```python
from build123d import *

# Parameters (mm, degrees)
SKETCH4_R           = 2.1
BOSS_EXTRUDE3_DEPTH = 1.2
SKETCH5_W           = 84.339489928
SKETCH5_H           = 2
BOSS_EXTRUDE4_DEPTH = 2.4
SKETCH6_R           = 2.1
BOSS_EXTRUDE5_DEPTH = 1.2


with BuildPart() as part:
    # Sketch4 → Boss-Extrude3 (new body)
    with BuildSketch(Plane(origin=(0, 0, 0), x_dir=(1, 0, 0), z_dir=(0, 1, 0))):
        Polygon((39.4127274, 47.640295112), (-2.757017564, 47.640295112), (-2.757017564, 45.640295112), (39.4127274, 0.640295112), align=None)
        with Locations((22.381300815, 25.64100497)):
            Circle(SKETCH4_R, mode=Mode.SUBTRACT)
        Polygon((81.582472364, 47.640295112), (39.4127274, 47.640295112), (39.4127274, 0.640295112), (81.582472364, 45.640295112), align=None)
        with Locations((56.444153985, 25.64100497)):
            Circle(SKETCH4_R, mode=Mode.SUBTRACT)
    extrude(amount=BOSS_EXTRUDE3_DEPTH)

    # Sketch5 → Boss-Extrude4 (add)
    with BuildSketch(Plane(origin=(0, 0, 0), x_dir=(-1, 0, 0), z_dir=(0, -1, 0))):
        with Locations((-39.4127274, 46.640295112)):
            Rectangle(SKETCH5_W, SKETCH5_H)
    extrude(amount=BOSS_EXTRUDE4_DEPTH)

    # Sketch6 → Boss-Extrude5 (add)
    with BuildSketch(Plane(origin=(0, -2.4, 0), x_dir=(-1, 0, 0), z_dir=(0, -1, 0))):
        Polygon((2.757017564, 47.640295112), (-81.582472364, 47.640295112), (-81.582472364, 45.640295112), (-39.4127274, 0.640295112), (2.757017564, 45.640295112), align=None)
        with Locations((-22.381300815, 25.64100497)):
            Circle(SKETCH6_R, mode=Mode.SUBTRACT)
        with Locations((-56.444153985, 25.64100497)):
            Circle(SKETCH6_R, mode=Mode.SUBTRACT)
    extrude(amount=BOSS_EXTRUDE5_DEPTH)


solid = part.part
```
Check sheet for the modelled part. Datum: model origin and axes. Units: mm. A direction names the side the tool comes from. Coordinates: 2 decimals unless noted, no trailing zeros. Order: outer loops, then holes, each group sorted by start corner. A loop starts at its lowest first (then second) coordinate and runs counter-clockwise, first axis right, second up. Notation, with made-up numbers: (13.25, -8) -> (72.25, -8) arc R24 cw to (72.25, 30) -> close; hole circle Ø1 at (85, -26.5). An arc over 180 degrees is marked (long way). Write item = value, one per line. Start each with the question number.
1) Mould release check, pull along Y, two halves, no side actions. Record for faces 1 (the cylindrical face through (58.447, 0.592, -26.272)), 2 (the flat face through (39, 0, -28)), 3 (the flat face through (40, -3.6, -35)): +Y half, -Y half, draft (parallel to the pull), parting line (faces both ways), or undercut.
2) Cross-section at A-A (z = -30). Enter the section's corners in (x, y).
3) Cross-section at B-B (x = 31). Enter the section's corners in (y, z).
4) Material ranges on L1, parallel to Y at x = 51, z = -14; L2, parallel to Z at x = 24, y = 0.2; L3, parallel to X at y = 0.4, z = -26, recorded low to high.
5) Cross-section at C-C (y = -0.9). Enter the section's corners in (x, z).
6) Go/stop test with flat-tipped pins: P1, Ø0.7, axis at x = 18.5, y = -1, coming from the +Z side; P2, Ø1.5, axis at x = 8.5, y = 0, coming from the +Z side. Record where each tip stops, or that it passes through.
7) Cross-section at D-D (z = -7.5). Enter the section's corners in (x, y).
8) Access from +Z, -Z, +X, -X, +Y, -Y to the whole of each face (thin tool, end or side, straight path). Record for faces 4 (the flat face through (60.793, -2.992, -23.455)), 5 (the flat face through (40, -1, -45.64)).
Ans:
q1.face_1 = draft
q1.face_2 = undercut
q1.face_3 = -Y half
q2.outline = (11.9, -3.6) -> (66.93, -3.6) -> (66.93, -2.4) -> (11.9, -2.4) -> close; (11.9, 0) -> (66.93, 0) -> (66.93, 1.2) -> (11.9, 1.2) -> close
q3.outline = (-3.6, -47.64) -> (1.2, -47.64) -> (1.2, -9.62) -> (0, -9.62) -> (0, -45.64) -> (-2.4, -45.64) -> (-2.4, -9.62) -> (-3.6, -9.62) -> close
q4.L1 = -3.6 to -2.4, 0 to 1.2
q4.L2 = -47.64 to -26.98, -24.3 to -17.09
q4.L3 = 15.65 to 20.31, 24.45 to 54.38, 58.51 to 63.18
q5.outline = (-2.76, -47.64) -> (81.58, -47.64) -> (81.58, -45.64) -> (-2.76, -45.64) -> close
q6.P1 = -45.64
q6.P2 = -32.83
q7.outline = (32.98, -3.6) -> (45.84, -3.6) -> (45.84, -2.4) -> (32.98, -2.4) -> close; (32.98, 0) -> (45.84, 0) -> (45.84, 1.2) -> (32.98, 1.2) -> close
q8.face_4 = +Z, +X, +Y, -Y
q8.face_5 = +Z, +X, -X
